from build123d import *

# Parameters (mm, degrees)
SKETCH2_R           = 30
BOSS_EXTRUDE1_DEPTH = 11.67
BOSS_EXTRUDE2_START = -57
SKETCH4_R           = 43.3
SKETCH4_R_2         = 30
BOSS_EXTRUDE2_DEPTH = 57
FILLET1_R           = 2


with BuildPart() as part:
    # Sketch2 → Boss-Extrude1 (new, symmetric)
    with BuildSketch(Plane.XY):
        with BuildLine():
            Line((-12.5, 120), (12.5, 120))
            ThreePointArc((12.5, 120), (20.236345621, 101.995330975), (23.643859133, 82.697455395))
            ThreePointArc((23.643859133, 82.697455395), (36.1, 62.527034153), (59.796167634, 61.824910351))
            ThreePointArc((59.796167634, 61.824910351), (78.212374881, 68.522854875), (97.673048454, 70.825317547))
            Line((97.673048454, 70.825317547), (110.173048454, 49.174682453))
            ThreePointArc((110.173048454, 49.174682453), (98.448720503, 33.4724761), (83.440026767, 20.872545044))
            ThreePointArc((83.440026767, 20.872545044), (72.2, 0), (83.440026767, -20.872545044))
            ThreePointArc((83.440026767, -20.872545044), (98.448720503, -33.4724761), (110.173048454, -49.174682453))
            Line((110.173048454, -49.174682453), (97.673048454, -70.825317547))
            ThreePointArc((97.673048454, -70.825317547), (78.212374881, -68.522854875), (59.796167634, -61.824910351))
            ThreePointArc((59.796167634, -61.824910351), (36.1, -62.527034153), (23.643859133, -82.697455395))
            ThreePointArc((23.643859133, -82.697455395), (20.236345621, -101.995330975), (12.5, -120))
            Line((12.5, -120), (-12.5, -120))
            ThreePointArc((-12.5, -120), (-20.236345621, -101.995330975), (-23.643859133, -82.697455395))
            ThreePointArc((-23.643859133, -82.697455395), (-36.1, -62.527034153), (-59.796167634, -61.824910351))
            ThreePointArc((-59.796167634, -61.824910351), (-78.212374881, -68.522854875), (-97.673048454, -70.825317547))
            Line((-97.673048454, -70.825317547), (-110.173048454, -49.174682453))
            ThreePointArc((-110.173048454, -49.174682453), (-98.448720503, -33.4724761), (-83.440026767, -20.872545044))
            ThreePointArc((-83.440026767, -20.872545044), (-72.2, 0), (-83.440026767, 20.872545044))
            ThreePointArc((-83.440026767, 20.872545044), (-98.448720503, 33.4724761), (-110.173048454, 49.174682453))
            Line((-110.173048454, 49.174682453), (-97.673048454, 70.825317547))
            ThreePointArc((-97.673048454, 70.825317547), (-78.212374881, 68.522854875), (-59.796167634, 61.824910351))
            ThreePointArc((-59.796167634, 61.824910351), (-36.1, 62.527034153), (-23.643859133, 82.697455395))
            ThreePointArc((-23.643859133, 82.697455395), (-20.236345621, 101.995330975), (-12.5, 120))
        make_face()
        Circle(SKETCH2_R, mode=Mode.SUBTRACT)
    extrude(amount=BOSS_EXTRUDE1_DEPTH, both=True)

    # Sketch3 → Cut-Revolve3 (revolve, cut)
    with BuildSketch(Plane(origin=(0, 0, 0), x_dir=(0, 0, -1), z_dir=(1, 0, 0))):
        with BuildLine():
            Line((-9.298765392, 121.603522868), (-9.298765392, 129.425144156))
            Line((-9.298765392, 129.425144156), (-28.94821126, 129.425144156))
            Line((-28.94821126, 129.425144156), (-28.94821126, 101.348727697))
            Line((-28.94821126, 101.348727697), (-11.67, 101.348727697))
            ThreePointArc((-11.67, 101.348727697), (-9.89359142, 111.406961181), (-9.298765392, 121.603522868))
        make_face()
    cut_revolve3 = revolve(axis=Axis((0, 0, 0), (0, 0, -1)), mode=Mode.SUBTRACT)

    # Mirror1: Cut-Revolve3 across plane
    add(cut_revolve3.mirror(Plane.XY), mode=Mode.SUBTRACT)

    # Sketch4 → Boss-Extrude2 (add)
    with BuildSketch(Plane.XY.offset(11.67).offset(BOSS_EXTRUDE2_START)):
        Circle(SKETCH4_R)
        Circle(SKETCH4_R_2, mode=Mode.SUBTRACT)
    extrude(amount=BOSS_EXTRUDE2_DEPTH)

    # Sketch5 → Revolve1 (revolve)
    with BuildSketch(Plane(origin=(0, 0, 0), x_dir=(0, 0, -1), z_dir=(1, 0, 0)), mode=Mode.PRIVATE) as revolve1_sk:
        Polygon((27.83, 43.3), (11.67, 43.3), (11.67, 52.31), align=None)
    revolve(revolve1_sk.sketch.rotate(Axis((0, 0, 0), (0, 0, 1)), 270), axis=Axis((0, 0, 0), (0, 0, 1)))

    # Fillet1
    fillet1_edges = [part.edges().sort_by_distance(p)[0] for p in [
        (-43.3, 0, -45.33),
    ]]
    fillet(fillet1_edges, radius=FILLET1_R)


solid = part.part
CAD build for the part. Positions are in the model's coordinates, mm. A direction names the side the tool comes from. Coordinates: 2 decimals unless noted, no trailing zeros. Write each loop counter-clockwise with the first axis right and the second up, starting at its lowest first coordinate (ties: lowest second). Pieces come first, ordered by that corner, then holes. Notation, with made-up numbers: M 7,-3 L 51,-3 A6 cw 51,4 Z; hole C 11.5,-14 d9. An arc over 180 degrees is marked long. Answer as a JSON object with one key per item and string values. Group by question number.
1) Saw through at A-A (y = 0). Write the cut outline in (x, z).
2) Wall check: line 1 (Y direction, x = 0, z = -25.5); line 2 (Y direction, x = 0, z = -13); line 3 (Z direction, x = -16.5, y = -99). Give the ranges that are in metal, low to high. Write a range as from..to.
3) Saw through at D-D (z = -34). Write the cut outline in (x, y), plus the area to 3 significant figures.
4) Pin check, flat tips, straight feed: pin 1 Ø5 at (y, z) = (-17, -2.5) entering from +X; pin 2 Ø5 at (x, y) = (-21, -65) entering from -Z; pin 3 Ø3 at (y, z) = (-60.5, 5) entering from +X. Stop position of each tip, or through.
5) Saw through at B-B (x = 0). Write the cut outline in (y, z).
6) Saw through at C-C (z = -1). Write the cut outline in (x, y).
7) Mould opens along X. For faces 5 (the face through (0, -120, 0)), 6 (the face through (78.48, -68.586, 0.163)), 7 (the face through (20.157, 102.259, 0.163)) say: +X half, -X half, draft (parallel to the pull), parting line (faces both ways), or undercut.
8) Tool access for faces 1 (the face through (-77.945, -68.459, 0.163)), 2 (the face through (-78.48, 68.586, 0.163)), 3 (the face through (-41, -44, -11.67)), 4 (the face through (98.637, 33.673, 0.163)): list every direction of +Z, -Z, +X, -X, +Y, -Y with a clear straight run to the whole face (end or side of a thin tool).
Values follow:
{
 "1": {"outline": "M -72.2,-11.67 L -52.31,-11.67 L -43.3,-27.83 L -43.3,-43.33 A2 ccw -41.3,-45.33 L -30,-45.33 L -30,11.67 L -72.2,11.67 Z; M 30,-45.33 L 41.3,-45.33 A2 ccw 43.3,-43.33 L 43.3,-27.83 L 52.31,-11.67 L 72.2,-11.67 L 72.2,11.67 L 30,11.67 Z"},
 "2": {"line 1": "y = -44.6..-30, 30..44.6", "line 2": "y = -51.57..-30, 30..51.57", "line 3": "z = -11.67..11.67"},
 "3": {"outline": "C 0,0 d86.6; hole C 0,0 d60", "area": "3,060 mm2"},
 "4": {"pin 1": "stops at x = 81.56", "pin 2": "stops at z = -11.67", "pin 3": "stops at x = 104.5"},
 "5": {"outline": "M -120,-9.31 A87.69 cw -101.35,-11.67 L -52.31,-11.67 L -43.3,-27.83 L -43.3,-43.33 A2 ccw -41.3,-45.33 L -30,-45.33 L -30,11.67 L -101.35,11.67 A87.69 cw -120,9.31 Z; M 30,-45.33 L 41.3,-45.33 A2 ccw 43.3,-43.33 L 43.3,-27.83 L 52.31,-11.67 L 101.35,-11.67 A87.69 cw 120,-9.31 L 120,9.31 A87.69 cw 101.35,11.67 L 30,11.67 Z"},
 "6": {"outline": "M -110.17,-49.17 L -97.67,-70.83 A85 ccw -59.8,-61.82 A25 cw -23.64,-82.7 A85 ccw -12.5,-120 L 12.5,-120 A85 ccw 23.64,-82.7 A25 cw 59.8,-61.82 A85 ccw 97.67,-70.83 L 110.17,-49.17 A85 ccw 83.44,-20.87 A25 cw 83.44,20.87 A85 ccw 110.17,49.17 L 97.67,70.83 A85 ccw 59.8,61.82 A25 cw 23.64,82.7 A85 ccw 12.5,120 L -12.5,120 A85 ccw -23.64,82.7 A25 cw -59.8,61.82 A85 ccw -97.67,70.83 L -110.17,49.17 A85 ccw -83.44,20.87 A25 cw -83.44,-20.87 A85 ccw Z; hole C 0,0 d60"},
 "7": {"face 5": "draft", "face 6": "undercut", "face 7": "+X half"},
 "8": {"face 1": "+Z, -Z, -Y", "face 2": "+Z, -Z, +Y", "face 3": "-Z", "face 4": "+Z, -Z, +X"}
}
